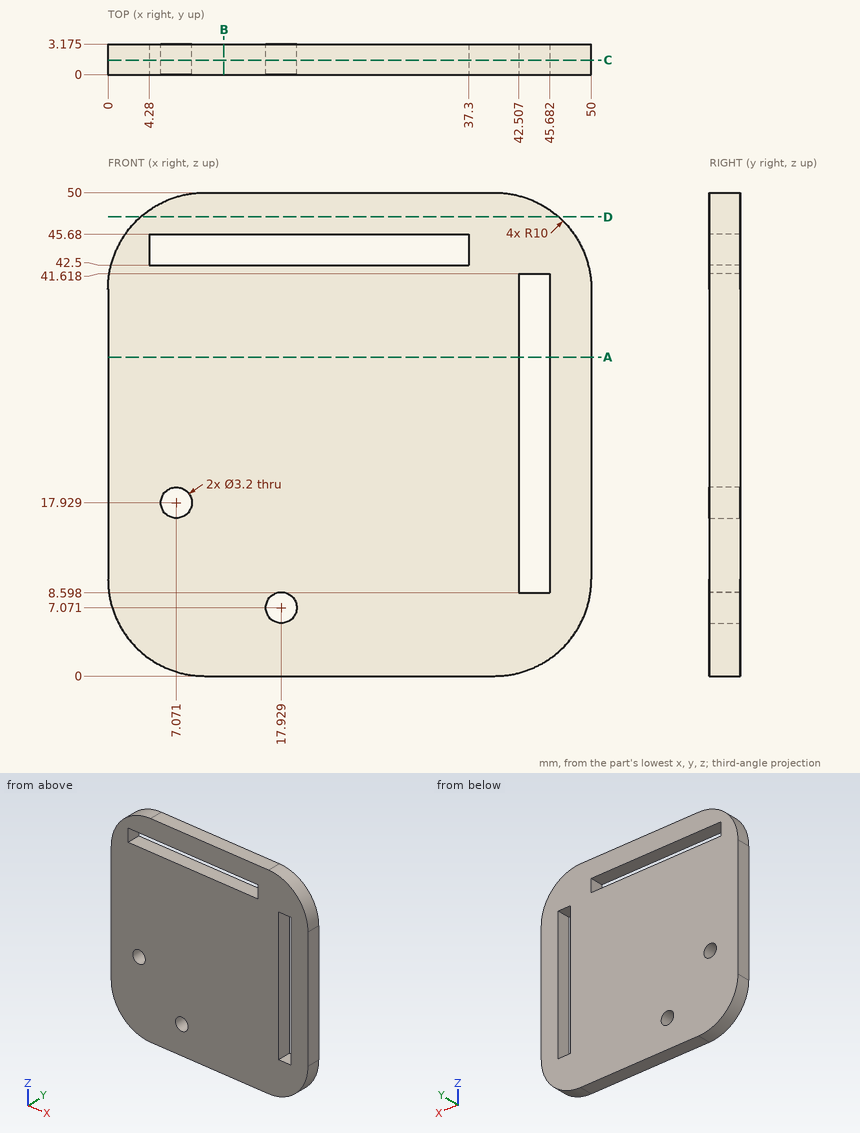
The figure shows three views and two pictorial views of one solid part (mm, origin at its lowest corner). Answer the questions. Give positions to 0.01 mm unless a question says otherwise; leave off trailing zeros. Order: outer loops, then holes, each group sorted by start corner. A loop starts at its lowest first (then second) coordinate and runs counter-clockwise, first axis right, second up. Notation, with made-up numbers: M 33.5,84.25 L 89.5,84.25 A24 cw 89.5,110.25 Z; hole C -17.75,-39.75 d1. An arc over 180 degrees is marked long. Return JSON: item names as keys, results as strings.
1) Section A-A, the plane z = 33 is taken. Write down the section's boundary in (x, y) (3 decimals), plus the area to 3 significant figures.
Resolved:
{"outline": "M 0,0 L 42.507,0 L 42.507,3.175 L 0,3.175 Z; M 45.682,0 L 50,0 L 50,3.175 L 45.682,3.175 Z", "area": "149 mm^2"}
2) Each of these flat-tipped pins is pushed along its axis until it touches: pin 1 (1.9 mm diameter, centred on x = 7.07, z = 17.93, fed in from -Y); pin 2 (1 mm diameter, centred on x = 44.5, y = 1.5, fed in from -Z) (3 decimals); pin 3 (2 mm diameter, centred on x = 6, z = 41.5, fed in from -Y); pin 4 (1 mm diameter, centred on y = 1.5, z = 44, fed in from -X). Where does it stop, or does it pass through?
Resolved:
{"pin 1": "through", "pin 2": "z = 0.835", "pin 3": "y = 0", "pin 4": "x = 0.63"}
3) Straight lines are drawn through the part: line 1 along Z through (x, y) = (12, 2.2); line 2 along X through (y, z) = (0.4, 23.5); line 3 along Z through (x, y) = (19, 1.6). For each, find the intervals that lie inside material, in ascending order. Write a range as [from, to].
Resolved:
{"line 1": "[0, 42.5], [45.68, 50]", "line 2": "[0, 42.51], [45.68, 50]", "line 3": "[0, 5.88], [8.26, 42.5], [45.68, 50]"}
4) Section B-B, the plane x = 12 is taken. Write down the section's boundary in (y, z) (3 decimals).
Resolved:
{"outline": "M 0,0 L 3.175,0 L 3.175,42.5 L 0,42.5 Z; M 0,45.68 L 3.175,45.68 L 3.175,50 L 0,50 Z"}
5) Section D-D, the plane z = 47.5 is taken. Write down the section's boundary in (x, y) (1 decimal).
Resolved:
{"outline": "M 3.4,0 L 46.6,0 L 46.6,3.2 L 3.4,3.2 Z"}
6) Section C-C, the plane y = 1.5 is taken. Write down the section's boundary in (x, z).
Resolved:
{"outline": "M 0,10 A10 ccw 10,0 L 40,0 A10 ccw 50,10 L 50,40 A10 ccw 40,50 L 10,50 A10 ccw 0,40 Z; hole M 4.28,42.5 L 37.3,42.5 L 37.3,45.68 L 4.28,45.68 Z; hole C 7.07,17.93 d3.2; hole C 17.93,7.07 d3.2; hole M 42.51,8.6 L 45.68,8.6 L 45.68,41.62 L 42.51,41.62 Z"}
